```python
from build123d import *

# Parameters (mm, degrees)
SKETCH_1_W          = 500
SKETCH_1_H          = 250
EXTRUDE_1_DEPTH     = 3.6
SKETCH_2_W          = 50
SKETCH_2_H          = 4
CUT_EXTRUDE_1_DEPTH = 3.6
SKETCH_3_W          = 4
SKETCH_3_H          = 50
SKETCH_3_H_2        = 41.448480175
CUT_EXTRUDE_2_DEPTH = 3.6


with BuildPart() as part:
    # 草图1 → 凸台-拉伸1 (new body)
    with BuildSketch(Plane.XY):
        Rectangle(SKETCH_1_W, SKETCH_1_H)
    extrude(amount=EXTRUDE_1_DEPTH)

    # 草图2 → 切除-拉伸1 (cut)
    with BuildSketch(Plane.XY.offset(3.6)):
        with Locations((0, 123)):
            Rectangle(SKETCH_2_W, SKETCH_2_H)
        with Locations((-110, 123)):
            Rectangle(SKETCH_2_W, SKETCH_2_H)
        with Locations((-210, 123)):
            Rectangle(SKETCH_2_W, SKETCH_2_H)
        with Locations((110, 123)):
            Rectangle(SKETCH_2_W, SKETCH_2_H)
        with Locations((210, 123)):
            Rectangle(SKETCH_2_W, SKETCH_2_H)
        with Locations((210, -123)):
            Rectangle(SKETCH_2_W, SKETCH_2_H)
        with Locations((110, -123)):
            Rectangle(SKETCH_2_W, SKETCH_2_H)
        with Locations((-210, -123)):
            Rectangle(SKETCH_2_W, SKETCH_2_H)
        with Locations((-110, -123)):
            Rectangle(SKETCH_2_W, SKETCH_2_H)
        with Locations((0, -123)):
            Rectangle(SKETCH_2_W, SKETCH_2_H)
    extrude(amount=-CUT_EXTRUDE_1_DEPTH, mode=Mode.SUBTRACT)

    # 草图3 → 切除-拉伸2 (cut)
    with BuildSketch(Plane.XY.offset(3.6)):
        with Locations((-248, 0)):
            Rectangle(SKETCH_3_W, SKETCH_3_H)
        with Locations((-248, 110)):
            Rectangle(SKETCH_3_W, SKETCH_3_H)
        with Locations((-248, -110)):
            Rectangle(SKETCH_3_W, SKETCH_3_H)
        with Locations((248, 4.275759912)):
            Rectangle(SKETCH_3_W, SKETCH_3_H_2)
        with Locations((248, -101.448480175)):
            Rectangle(SKETCH_3_W, SKETCH_3_H)
        with Locations((248, 110)):
            Rectangle(SKETCH_3_W, SKETCH_3_H)
    extrude(amount=-CUT_EXTRUDE_2_DEPTH, mode=Mode.SUBTRACT)


solid = part.part
```
Design review of the part built by this model. Coordinates are the model's own, in mm. Round coordinates to 2 decimals unless told otherwise and drop trailing zeros. Write each loop counter-clockwise with the first axis right and the second up, starting at its lowest first coordinate (ties: lowest second). Pieces come first, ordered by that corner, then holes.
Item 1: We need section A-A on x = -2.5. Write out the cut boundary in (y, z).
Item 2: For probe 1 along Y at (x, z) = (3, 2.7); probe 2 along X at (y, z) = (-22.5, 2.8); probe 3 along X at (y, z) = (12, 0.55), list the stretches that pass through material, from the lowest coordinate up.
Item 3: We need section B-B on y = -11.5. Write out the cut boundary in (x, z).
Item 4: Clearance check with flat-ended pins moving along their axes: pin 1 Ø2 at (x, z) = (0, 0.5) entering from -Y; pin 2 Ø8 at (x, y) = (43.5, 47.5) entering from -Z; pin 3 Ø2 at (y, z) = (86.5, 3) entering from +X. State where each tip first meets the part, or that it passes through.
Returned:
1. outline: (-121, 0) - (121, 0) - (121, 3.6) - (-121, 3.6) - close
2. probe 1: y = -121 to 121
2. probe 2: x = -246 to 250
2. probe 3: x = -246 to 246
3. outline: (-246, 0) - (246, 0) - (246, 3.6) - (-246, 3.6) - close
4. pin 1: stops at y = -121
4. pin 2: stops at z = 0
4. pin 3: stops at x = 246
